Source: three-view drawing plus pictorial views. Frame: mm from the lowest corner of the part. A direction names the side the tool comes from. Give positions to 0.01 mm unless a question says otherwise; leave off trailing zeros. Loops run counter-clockwise (first coordinate to the right, second up) from the corner with the lowest first, then second, coordinate; pieces in that order, holes last.
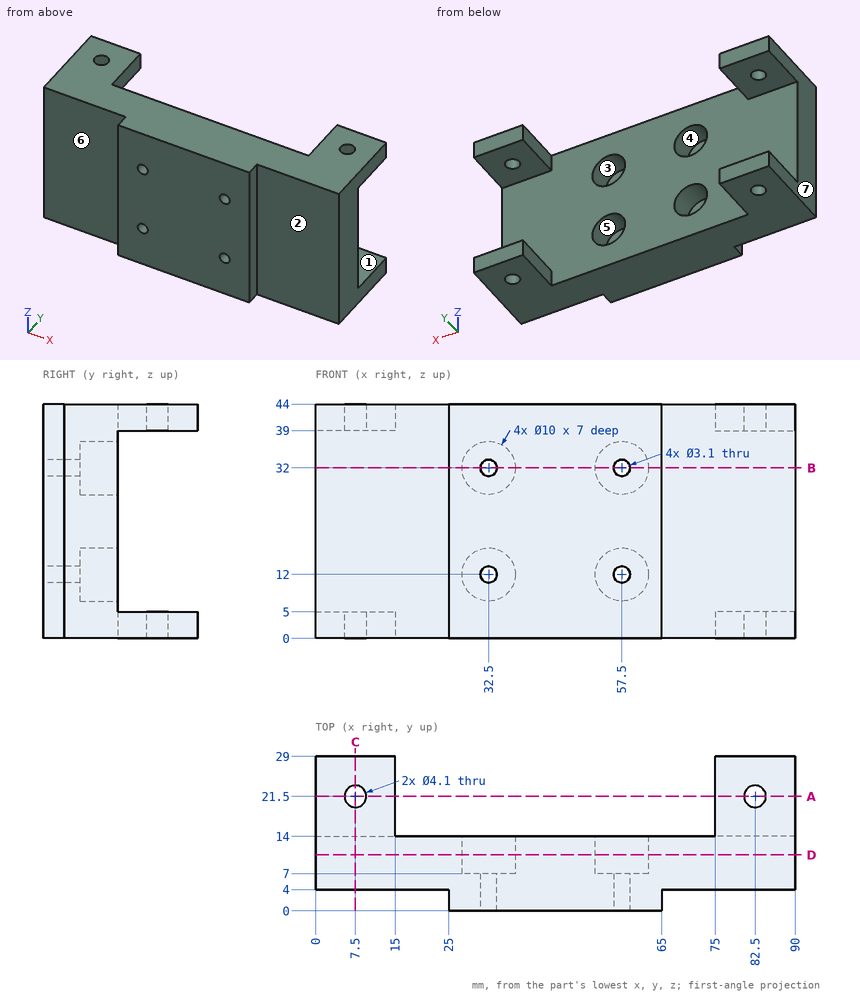
1) Contact query for flat-ended pins moving along their axis: P1, Ø3, axis at x = 55.5, z = 30.5, coming from the +Y side; P2, Ø7.5, axis at x = 82, z = 13, coming from the -Y side; P3, Ø3, axis at y = 1, z = 22, coming from the +X side. Output: stop coordinate, or through.
Checks:
P1: stops at y = 7
P2: stops at y = 4
P3: stops at x = 65
2) Reachability of the marked faces 1, 2 and 3 from +Z, -Z, +X, -X, +Y, -Y: full face, straight path, thin tool, end or side. Return the list, or none.
Checks:
face 1: +X, -X, +Y
face 2: +Z, -Z, +X, -Y
face 3: +Y
3) Pull-direction query (X, two-part tool) for the marked faces 4, 5, 6 and 7; classes: released by +X, released by -X, zero draft, split by the parting line, or undercut.
Checks:
face 4: undercut
face 5: undercut
face 6: zero draft
face 7: released by -X
4) Ray query, probe 1 along Z at (x, y) = (32.5, 3.25); probe 2 along X at (y, z) = (2.75, 12); probe 3 along X at (y, z) = (5, 12). Return the intervals inside material, ascending.
Checks:
probe 1: z = 0 to 10.45, 13.55 to 30.45, 33.55 to 44
probe 2: x = 25 to 30.95, 34.05 to 55.95, 59.05 to 65
probe 3: x = 0 to 30.95, 34.05 to 55.95, 59.05 to 90
5) Cut plane B-B (z = 32). Return loops of the section in (x, y).
Checks:
outline: (0, 4) - (25, 4) - (25, 0) - (30.95, 0) - (30.95, 7) - (27.5, 7) - (27.5, 14) - (0, 14) - close; (34.05, 0) - (55.95, 0) - (55.95, 7) - (52.5, 7) - (52.5, 14) - (37.5, 14) - (37.5, 7) - (34.05, 7) - close; (59.05, 0) - (65, 0) - (65, 4) - (90, 4) - (90, 14) - (62.5, 14) - (62.5, 7) - (59.05, 7) - close
6) Cut plane D-D (y = 10.5). Return loops of the section in (x, z).
Checks:
outline: (0, 0) - (90, 0) - (90, 44) - (0, 44) - close; hole circle Ø10 at (32.5, 12); hole circle Ø10 at (32.5, 32); hole circle Ø10 at (57.5, 12); hole circle Ø10 at (57.5, 32)
7) Cut plane C-C (x = 7.5). Return loops of the section in (y, z), and give its area (3 significant figures).
Checks:
outline: (4, 0) - (19.45, 0) - (19.45, 5) - (14, 5) - (14, 39) - (19.45, 39) - (19.45, 44) - (4, 44) - close; (23.55, 0) - (29, 0) - (29, 5) - (23.55, 5) - close; (23.55, 39) - (29, 39) - (29, 44) - (23.55, 44) - close
area: 549 mm2
8) Cut plane A-A (y = 21.5). State how many separate pieces and enclosed holes the cut face has, and give its area (3 significant figures).
Checks:
separate pieces: 8
enclosed holes: 0
area: 218 mm2
